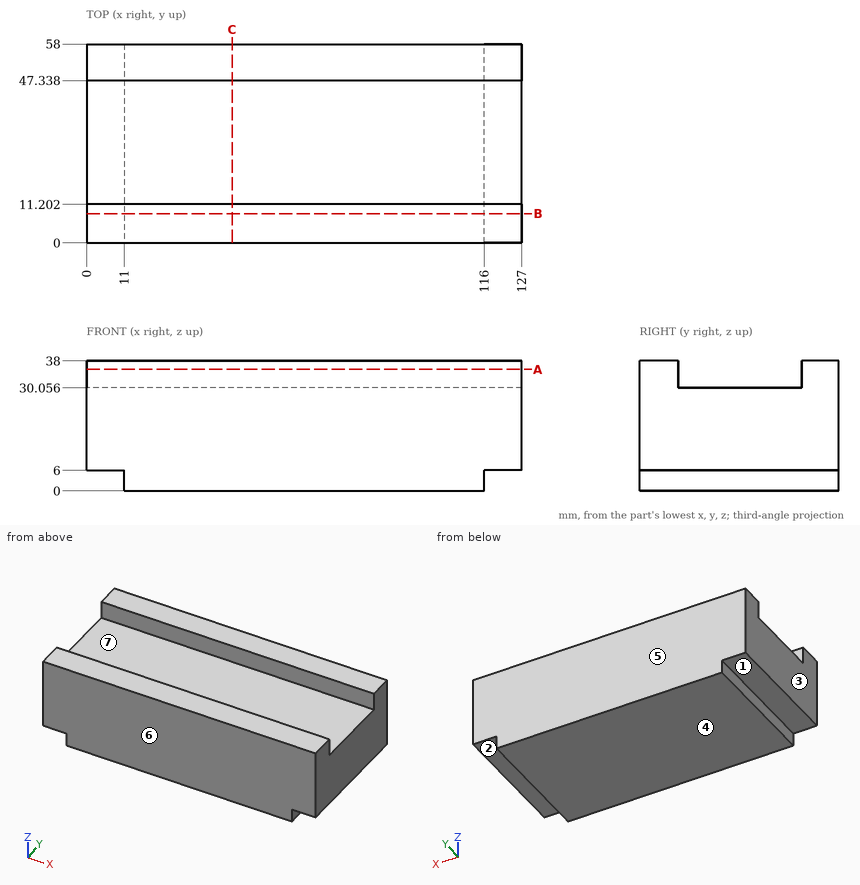
Answer from the drawing. Dimensions are ordinates in mm from the lowest x, y and z of the part. A direction names the side the tool comes from. Coordinates: 2 decimals unless noted, no trailing zeros. Order: outer loops, then holes, each group sorted by start corner. A loop starts at its lowest first (then second) coordinate and runs counter-clockwise, first axis right, second up. Notation, with made-up numbers: (-2, 57) - (5, 57) arc R10 ccw to (5, 64) - close; hole circle Ø6 at (-34.75, 10). An arc over 180 degrees is marked (long way). Put each result on its own line as item: value. Start each with the question number.
1) Find section B-B (y = 8.5). Give the vertices of the cut face in (x, z), plus the area to 3 significant figures.
2) For a pull along Y with two mould halves and no side action, classify the marked faces 4, 5, 6 and 7 as released by +Y, released by -Y, zero draft, split by the parting line, or undercut.
3) Flat-ended cylindrical pins translate along their axes: pin 1 (1.8 mm diameter, centred on y = 21, z = 3.5, fed in from -X); pin 2 (1.8 mm diameter, centred on y = 40.5, z = 2, fed in from +X); pin 3 (5.5 mm diameter, centred on x = 119.5, y = 39.5, fed in from -Z). Find the tip coordinate at first contact, or state that the pin passes through.
4) For the marked faces 1, 2 and 3, determine the directions among +Z, -Z, +X, -X, +Y, -Y from which every point of the face is accessible in a straight line to the end or side of a thin tool.
5) Find section A-A (z = 35.5). Give the vertices of the cut face in (x, y), plus the area to 3 significant figures.
6) Find section C-C (x = 42.5). Give the vertices of the cut face in (y, z), plus the area to 3 significant figures.
7) Find the intervals of material crossed by line 1 (Y direction, x = 120.5, z = 34.5); line 2 (X direction, y = 21, z = 3.5); line 3 (Z direction, x = 22.5, y = 45), in increasing order. Write a range as from..to.
Results list:
1. outline: (0, 6) - (11, 6) - (11, 0) - (116, 0) - (116, 6) - (127, 6) - (127, 38) - (0, 38) - close
1. area: 4,690 mm^2
2. face 4: zero draft
2. face 5: released by +Y
2. face 6: released by -Y
2. face 7: undercut
3. pin 1: stops at x = 11
3. pin 2: stops at x = 116
3. pin 3: stops at z = 6
4. face 1: -Z, -X, +Y, -Y
4. face 2: -Z, +X, +Y, -Y
4. face 3: +Z, -Z, -X, +Y, -Y
5. outline: (0, 0) - (127, 0) - (127, 11.2) - (0, 11.2) - close; (0, 47.34) - (127, 47.34) - (127, 58) - (0, 58) - close
5. area: 2,780 mm^2
6. outline: (0, 0) - (58, 0) - (58, 38) - (47.34, 38) - (47.34, 30.06) - (11.2, 30.06) - (11.2, 38) - (0, 38) - close
6. area: 1,920 mm^2
7. line 1: y = 0..11.2, 47.34..58
7. line 2: x = 11..116
7. line 3: z = 0..30.06
